Part model, mm, in its own coordinate system. Face numbers are marked on the shaded views. Coordinates: 2 decimals unless noted, no trailing zeros. Write each loop counter-clockwise with the first axis right and the second up, starting at its lowest first coordinate (ties: lowest second). Pieces come first, ordered by that corner, then holes. Notation, with made-up numbers: (52, 23.5) - (62, 23.5) arc R20 cw to (62, 49.5) - close; hole circle Ø2 at (18.5, 44.25). An arc over 180 degrees is marked (long way). Use a Markdown table: item, result.
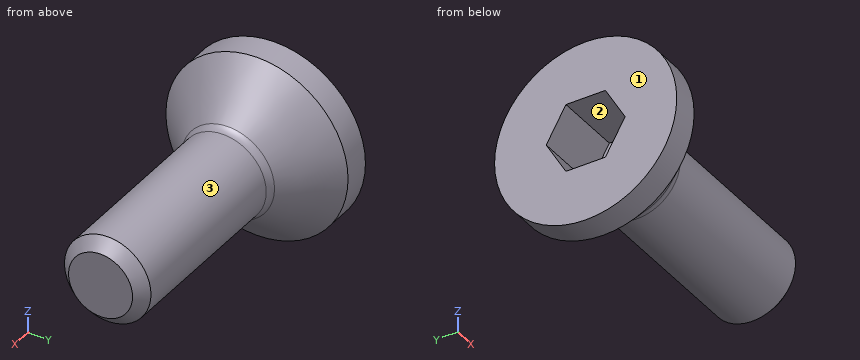
```python
from build123d import *

# Parameters (mm, degrees)
CUT_EXTRUDE1_DEPTH = 1.5


with BuildPart() as part:
    # Sketch1 → Revolve1 (revolve)
    with BuildSketch(Plane.XY):
        with BuildLine():
            Line((1.774861053, 0.95), (5.752512627, 0.95))
            Line((5.752512627, 0.95), (6, 0.702512627))
            Line((6, 0.702512627), (6, 0))
            Line((6, 0), (0, 0))
            Line((0, 0), (0, 2))
            Line((0, 2), (0.6, 2))
            Line((0.6, 2), (1.6, 1.0213282))
            ThreePointArc((1.6, 1.0213282), (1.680436347, 0.968517873), (1.774861053, 0.95))
        make_face()
    revolve(axis=Axis((0, 0, 0), (-1, 0, 0)))

    # Sketch2 → Cut-Extrude1 (cut)
    with BuildSketch(Plane.ZY):
        Polygon((0.75, 0.433012702), (0, 0.866025404), (-0.75, 0.433012702), (-0.75, -0.433012702), (0, -0.866025404), (0.75, -0.433012702), align=None)
    extrude(amount=-CUT_EXTRUDE1_DEPTH, mode=Mode.SUBTRACT)


solid = part.part
```
Item 1: Band-saw the part on C-C, the plane x = 2.25. Give the cut face in (y, z).
From the geometry:
| item | result |
|---|---|
| outline | circle Ø1.9 at (0, 0) |
Item 2: Drop flat-ended pins along their axis: P1, Ø0.5, axis at y = -0.5, z = 0, coming from the -X side; P2, Ø2, axis at x = 2, y = 1.5, coming from the +Z side. Give the stop position or say it passes through.
From the geometry:
| item | result |
|---|---|
| P1 | x = 1.5 |
| P2 | z = 1.09 |
Item 3: Drill centre lines: probe 1 along X at (y, z) = (-0.2, -0.15); probe 2 along Z at (x, y) = (4.5, -0.05); probe 3 along X at (y, z) = (-0.8, -1.3). Where is each one in solid material? Low to high.
From the geometry:
| item | result |
|---|---|
| probe 1 | 1.5 to 6 |
| probe 2 | -0.95 to 0.95 |
| probe 3 | 0 to 1.08 |
Item 4: Band-saw the part on B-B, the plane x = 0.8. Give the cut face in (y, z).
From the geometry:
| item | result |
|---|---|
| outline | circle Ø3.61 at (0, 0); hole (-0.87, 0) - (-0.43, -0.75) - (0.43, -0.75) - (0.87, 0) - (0.43, 0.75) - (-0.43, 0.75) - close |
Item 5: Band-saw the part on A-A, the plane y = 0. Give the cut face in (x, z), then the cut area to 3 significant figures.
From the geometry:
| item | result |
|---|---|
| outline | (0, -2) - (0.6, -2) - (1.6, -1.02) arc R0.25 cw to (1.77, -0.95) - (5.75, -0.95) - (6, -0.7) - (6, 0.7) - (5.75, 0.95) - (1.77, 0.95) arc R0.25 cw to (1.6, 1.02) - (0.6, 2) - (0, 2) - (0, 0.75) - (1.5, 0.75) - (1.5, -0.75) - (0, -0.75) - close |
| area | 11.5 mm^2 |
Item 6: Two-plate mould, pull along Y, no slides. Class the marked faces 1, 2 and 3: pulls with the +Y half, pulls with the -Y half, needs draft (parallel to the pull), parting line crosses it, or undercut.
From the geometry:
| item | result |
|---|---|
| face 1 | needs draft |
| face 2 | undercut |
| face 3 | parting line crosses it |
